from build123d import *

# Parameters (mm, degrees)
SKETCH1_W                = 60
SKETCH1_H                = 22
BOSS_EXTRUDE1_DEPTH      = 54
SKETCH2_W                = 40
SKETCH2_H                = 18
CUT_EXTRUDE1_DEPTH       = 54
CUT_EXTRUDE1_DEPTH_BACK  = 54
CUT_EXTRUDE2_DEPTH       = 12.8
SKETCH4_W                = 120
SKETCH4_H                = 180
CUT_EXTRUDE3_DEPTH       = 54
CUT_EXTRUDE3_DEPTH_BACK  = 54
SKETCH5_W                = 96
SKETCH5_H                = 64
CUT_EXTRUDE4_DEPTH       = 30
CUT_EXTRUDE4_DEPTH_BACK  = 30
SKETCH6_R                = 2.75
CUT_EXTRUDE5_DEPTH       = 15
SKETCH7_R                = 1.222222222
CUT_EXTRUDE6_DEPTH       = 15
SKETCH8_R                = 2.75
CUT_EXTRUDE7_DEPTH       = 30
CUT_EXTRUDE7_DEPTH_BACK  = 30
CUT_EXTRUDE8_DEPTH       = 50
SKETCH10_R               = 2.75
CUT_EXTRUDE9_DEPTH       = 15
SKETCH11_R               = 1.222222222
CUT_EXTRUDE10_DEPTH      = 15
SKETCH12_R               = 1.7
CUT_EXTRUDE11_DEPTH      = 3.2
CUT_EXTRUDE11_DEPTH_BACK = 3.2
SKETCH13_R               = 1.7
CUT_EXTRUDE12_DEPTH      = 3.2
CUT_EXTRUDE12_DEPTH_BACK = 3.2
CUT_EXTRUDE13_DEPTH      = 2.75
CUT_EXTRUDE13_DEPTH_BACK = 2.75
CUT_EXTRUDE14_DEPTH      = 2.75
CUT_EXTRUDE14_DEPTH_BACK = 2.75
BOSS_EXTRUDE2_DEPTH      = 2.909090909
BOSS_EXTRUDE2_DEPTH_BACK = 2.909090909
BOSS_EXTRUDE3_DEPTH      = 4.571428571
BOSS_EXTRUDE3_DEPTH_BACK = 4.571428571


with BuildPart() as part:
    # Sketch1 → Boss-Extrude1 (new body)
    with BuildSketch(Plane.XY):
        Rectangle(SKETCH1_W, SKETCH1_H)
    extrude(amount=-BOSS_EXTRUDE1_DEPTH)

    # Sketch2 → Cut-Extrude1 (cut, two sides)
    with BuildSketch(Plane.XY) as cut_extrude1_sk:
        with Locations((0, -2)):
            Rectangle(SKETCH2_W, SKETCH2_H)
    extrude(amount=CUT_EXTRUDE1_DEPTH, mode=Mode.SUBTRACT)
    extrude(cut_extrude1_sk.sketch, amount=-CUT_EXTRUDE1_DEPTH_BACK, mode=Mode.SUBTRACT)

    # Sketch3 → Cut-Extrude2 (cut)
    with BuildSketch(Plane.XY.offset(-21.56)):
        Polygon((-12, 11.66), (-11.410511777, 9.46), (11.410511777, 9.46), (12, 11.66), align=None)
    extrude(amount=-CUT_EXTRUDE2_DEPTH, mode=Mode.SUBTRACT)

    # Sketch4 → Cut-Extrude3 (cut, two sides)
    with BuildSketch(Plane(origin=(0, 0, 0), x_dir=(-1, 0, 0), z_dir=(0, 1, 0))) as cut_extrude3_sk:
        with Locations((0, -30)):
            Rectangle(SKETCH4_W, SKETCH4_H)
        Polygon((30, -54), (30, 0), (20, 0), (20, -17.6), (-20, -17.6), (-20, 0), (-30, 0), (-30, -54), (-20, -54), (-20, -38.6), (20, -38.6), (20, -54), align=None, mode=Mode.SUBTRACT)
    extrude(amount=CUT_EXTRUDE3_DEPTH, mode=Mode.SUBTRACT)
    extrude(cut_extrude3_sk.sketch, amount=-CUT_EXTRUDE3_DEPTH_BACK, mode=Mode.SUBTRACT)

    # Sketch5 → Cut-Extrude4 (cut, two sides)
    with BuildSketch(Plane(origin=(0, 0, 0), x_dir=(0, 0, -1), z_dir=(1, 0, 0))) as cut_extrude4_sk:
        with Locations((16, 0)):
            Rectangle(SKETCH5_W, SKETCH5_H)
        with BuildLine():
            Line((11, -11), (43, -11))
            ThreePointArc((43, -11), (54, 0), (43, 11))
            Line((43, 11), (11, 11))
            ThreePointArc((11, 11), (0, 0), (11, -11))
        make_face(mode=Mode.SUBTRACT)
    extrude(amount=CUT_EXTRUDE4_DEPTH, mode=Mode.SUBTRACT)
    extrude(cut_extrude4_sk.sketch, amount=-CUT_EXTRUDE4_DEPTH_BACK, mode=Mode.SUBTRACT)

    # Sketch6 → Cut-Extrude5 (cut)
    with BuildSketch(Plane(origin=(-24.7, 0, 0), x_dir=(0, 0, -1), z_dir=(1, 0, 0))):
        with BuildLine():
            Line((43, -11.5), (43, -38))
            Line((43, -38), (63.2, -38))
            Line((63.2, -38), (63.2, 41))
            Line((63.2, 41), (48.065075259, 41))
            Line((48.065075259, 41), (34.727592296, 7.98857126))
            ThreePointArc((34.727592296, 7.98857126), (32.414194185, -4.493407978), (43, -11.5))
        make_face()
        with Locations((43, 0)):
            Circle(SKETCH6_R, mode=Mode.SUBTRACT)
    extrude(amount=-CUT_EXTRUDE5_DEPTH, mode=Mode.SUBTRACT)

    # Sketch7 → Cut-Extrude6 (cut)
    with BuildSketch(Plane(origin=(-24.7, 0, 0), x_dir=(0, 0, -1), z_dir=(1, 0, 0))):
        with Locations((43, 0)):
            Circle(SKETCH7_R)
    extrude(amount=-CUT_EXTRUDE6_DEPTH, mode=Mode.SUBTRACT)

    # Sketch8 → Cut-Extrude7 (cut, two sides)
    with BuildSketch(Plane(origin=(0, 0, 0), x_dir=(0, 0, -1), z_dir=(1, 0, 0))) as cut_extrude7_sk:
        with Locations((11, 0)):
            Circle(SKETCH8_R)
    extrude(amount=CUT_EXTRUDE7_DEPTH, mode=Mode.SUBTRACT)
    extrude(cut_extrude7_sk.sketch, amount=-CUT_EXTRUDE7_DEPTH_BACK, mode=Mode.SUBTRACT)

    # Sketch9 → Cut-Extrude8 (cut)
    with BuildSketch(Plane(origin=(-25, 0, 0), x_dir=(0, 0, -1), z_dir=(1, 0, 0))):
        with BuildLine():
            Line((-2.2, 26), (-2.2, -33))
            Line((-2.2, -33), (11, -33))
            Line((11, -33), (11, -11.5))
            ThreePointArc((11, -11.5), (21.585805815, -4.493407978), (19.272407704, 7.98857126))
            Line((19.272407704, 7.98857126), (11.995318128, 26))
            Line((11.995318128, 26), (-2.2, 26))
        make_face()
    extrude(amount=CUT_EXTRUDE8_DEPTH, mode=Mode.SUBTRACT)

    # Sketch10 → Cut-Extrude9 (cut)
    with BuildSketch(Plane(origin=(24.7, 0, 0), x_dir=(0, 0, -1), z_dir=(1, 0, 0))):
        with BuildLine():
            Line((43, -19.032866311), (43, -38))
            Line((43, -38), (63.2, -38))
            Line((63.2, -38), (63.2, 41))
            Line((63.2, 41), (48.065075259, 41))
            Line((48.065075259, 41), (34.727592296, 7.98857126))
            ThreePointArc((34.727592296, 7.98857126), (31.646049671, -1.826967959), (37.651162791, -10.180370352))
            ThreePointArc((37.651162791, -10.180370352), (41.558961032, -13.861388181), (43, -19.032866311))
        make_face()
        with Locations((43, 0)):
            Circle(SKETCH10_R, mode=Mode.SUBTRACT)
    extrude(amount=CUT_EXTRUDE9_DEPTH, mode=Mode.SUBTRACT)

    # Sketch11 → Cut-Extrude10 (cut)
    with BuildSketch(Plane(origin=(24.7, 0, 0), x_dir=(0, 0, -1), z_dir=(1, 0, 0))):
        with Locations((43, 0)):
            Circle(SKETCH11_R)
    extrude(amount=CUT_EXTRUDE10_DEPTH, mode=Mode.SUBTRACT)

    # Sketch12 → Cut-Extrude11 (cut, two sides)
    with BuildSketch(Plane.XY.offset(-27)) as cut_extrude11_sk:
        Polygon((-30, -6.2), (-28, -6.2), (-28, -11), (-20, -11), (-20, -3.8), (-30, -3.8), align=None)
        with Locations((-22.5, -7)):
            Circle(SKETCH12_R, mode=Mode.SUBTRACT)
    extrude(amount=CUT_EXTRUDE11_DEPTH, mode=Mode.SUBTRACT)
    extrude(cut_extrude11_sk.sketch, amount=-CUT_EXTRUDE11_DEPTH_BACK, mode=Mode.SUBTRACT)

    # Sketch13 → Cut-Extrude12 (cut, two sides)
    with BuildSketch(Plane.XY.offset(-27)) as cut_extrude12_sk:
        Polygon((20, -11), (28, -11), (28, -6.2), (30, -6.2), (30, -3.8), (20, -3.8), align=None)
        with Locations((22.5, -7)):
            Circle(SKETCH13_R, mode=Mode.SUBTRACT)
    extrude(amount=CUT_EXTRUDE12_DEPTH, mode=Mode.SUBTRACT)
    extrude(cut_extrude12_sk.sketch, amount=-CUT_EXTRUDE12_DEPTH_BACK, mode=Mode.SUBTRACT)

    # Sketch14 → Cut-Extrude13 (cut, two sides)
    with BuildSketch(Plane(origin=(0, 0, 0), x_dir=(-1, 0, 0), z_dir=(0, 1, 0))) as cut_extrude13_sk:
        Polygon((-28.333333333, -45.75), (-30, -43), (-30, -45.75), align=None)
    extrude(amount=CUT_EXTRUDE13_DEPTH, mode=Mode.SUBTRACT)
    extrude(cut_extrude13_sk.sketch, amount=-CUT_EXTRUDE13_DEPTH_BACK, mode=Mode.SUBTRACT)

    # Sketch15 → Cut-Extrude14 (cut, two sides)
    with BuildSketch(Plane(origin=(0, 0, 0), x_dir=(-1, 0, 0), z_dir=(0, 1, 0))) as cut_extrude14_sk:
        Polygon((30, -45.75), (30, -43), (28.333333333, -45.75), align=None)
    extrude(amount=CUT_EXTRUDE14_DEPTH, mode=Mode.SUBTRACT)
    extrude(cut_extrude14_sk.sketch, amount=-CUT_EXTRUDE14_DEPTH_BACK, mode=Mode.SUBTRACT)

    # Sketch16 → Boss-Extrude2 (add, two sides)
    with BuildSketch(Plane.XY.offset(-27)) as boss_extrude2_sk:
        with BuildLine():
            Line((-23.4, -11), (23.4, -11))
            ThreePointArc((23.4, -11), (25.945584412, -9.945584412), (27, -7.4))
            Line((27, -7.4), (27, -5))
            Line((27, -5), (24.2, -5))
            Line((24.2, -5), (24.2, -7))
            ThreePointArc((24.2, -7), (22.5, -8.7), (20.8, -7))
            Line((20.8, -7), (-20.8, -7))
            ThreePointArc((-20.8, -7), (-22.5, -8.7), (-24.2, -7))
            Line((-24.2, -7), (-24.2, -5))
            Line((-24.2, -5), (-27, -5))
            Line((-27, -5), (-27, -7.4))
            ThreePointArc((-27, -7.4), (-25.945584412, -9.945584412), (-23.4, -11))
        make_face()
    extrude(amount=BOSS_EXTRUDE2_DEPTH)
    extrude(boss_extrude2_sk.sketch, amount=-BOSS_EXTRUDE2_DEPTH_BACK)

    # Sketch17 → Boss-Extrude3 (add, two sides)
    with BuildSketch(Plane.XY.offset(-27)) as boss_extrude3_sk:
        with BuildLine():
            Line((-19.379616013, -11), (19.379616013, -11))
            ThreePointArc((19.379616013, -11), (19.567915266, -10.867404682), (19.506538526, -10.645433911))
            ThreePointArc((19.506538526, -10.645433911), (18.409986139, -9.349848212), (17.843015997, -7.75))
            Line((17.843015997, -7.75), (-17.843015997, -7.75))
            ThreePointArc((-17.843015997, -7.75), (-18.409986139, -9.349848212), (-19.506538526, -10.645433911))
            ThreePointArc((-19.506538526, -10.645433911), (-19.567915266, -10.867404682), (-19.379616013, -11))
        make_face()
    extrude(amount=BOSS_EXTRUDE3_DEPTH)
    extrude(boss_extrude3_sk.sketch, amount=-BOSS_EXTRUDE3_DEPTH_BACK)


solid = part.part
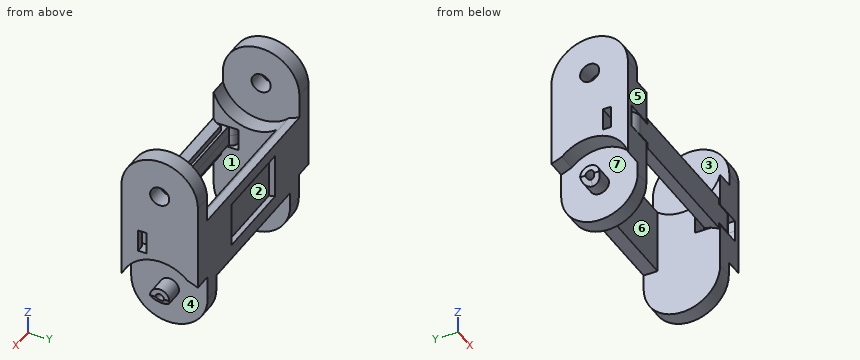
Here's how the part is built. I have some questions about the finished solid (model axes, mm). Face numbers are marked on the shaded views. A direction names the side the tool comes from. Coordinates: 2 decimals unless noted, no trailing zeros. Loops run counter-clockwise (first coordinate to the right, second up) from the corner with the lowest first, then second, coordinate; pieces in that order, holes last.
1. I need wall thicknesses on L1, parallel to Z at x = 27.45, y = 0; L2, parallel to X at y = -8.5, z = -39.5; L3, parallel to Y at x = -10, z = -30. Which ranges of each line are inside material? Lowest first, please.
2. If we mould it in two halves opening along Z, with no side actions, what happens to the marked faces 1 and 2? For each: pulls with the +Z half, pulls with the -Z half, needs draft (parallel to the pull), parting line crosses it, or undercut.
3. Imagine slicing it at A-A, the plane z = -25.5. Count the separate pieces of the cut face and the enclosed holes in it, and give its area (3 significant figures).
4. Imagine slicing it at C-C, the plane y = 4. Please give me the cut outline in (x, z), and give its area (3 significant figures).
5. For the marked faces 3, 4, 5, 6 and 7, which set-ups out of +Z, -Z, +X, -X, +Y, -Y let a thin tool reach every point of the face, with its end or its side?
6. Imagine slicing it at D-D, the plane z = -47. Please give me the cut outline in (x, y).
7. Imagine slicing it at B-B, the plane x = 22.5. Please give me the cut outline in (y, z).
8. For P1, Ø3, axis at x = -9, y = 9, coming from the -Z side; P2, Ø1.8, axis at x = 8.5, y = -9, coming from the -Z side; P3, Ø2, axis at x = 10, y = 5.5, coming from the -Z side; P4, Ø1.2, axis at x = 2.5, y = 10.5, coming from the +Z side, each with a flat end and sliding along its axis, tell me the tip position at first contact or that it passes through.
Taken from the geometry:
1. L1: z = -45.75 to -44.22, -41.78 to -40.25, -31.5 to -13.75, -8.25 to 0
1. L2: x = -24.7 to -20, 20 to 24.7
1. L3: y = -11 to -7.75, 7 to 9.46
2. face 1: needs draft
2. face 2: undercut
3. separate pieces: 4
3. enclosed holes: 0
3. area: 670 mm2
4. outline: (-30, -32.22) - (-24.7, -32.22) - (-24.7, -53.25) - (-20, -53.25) - (-20, -21.78) - (-25, -21.78) - (-25, -0.75) - (-30, -0.75) - close; (20, -53.25) - (24.7, -53.25) - (24.7, -32.22) - (30, -32.22) - (30, -0.75) - (25, -0.75) - (25, -21.78) - (20, -21.78) - close
4. area: 617 mm2
5. face 3: +Z
5. face 4: +X
5. face 5: +Z, -Z, +X, -X, -Y
5. face 6: +Z, -Z
5. face 7: -X
6. outline: (-24.7, -10.25) - (-20, -10.25) - (-20, 10.25) - (-24.7, 10.25) - close; (20, -10.25) - (24.7, -10.25) - (24.7, 10.25) - (20, 10.25) - close
7. outline: (-11, -43) arc R11 ccw to (11, -43) - (11, -18.06) - (7.99, -19.27) arc R11.5 cw to (-11, -14.35) - (-11, -23.8) - (-8.7, -23.8) - (-8.7, -24.09) - (-11, -24.09) - (-11, -29.91) - (-8.7, -29.91) - (-8.7, -30.2) - (-11, -30.2) - close; hole (-5.3, -30.2) - (-3.8, -30.2) - (-3.8, -23.8) - (-5.3, -23.8) - close
8. P1: stops at z = -38.6
8. P2: stops at z = -31.57
8. P3: passes through
8. P4: stops at z = -18.06
